from build123d import *

# Parameters (mm, degrees)
SKETCH1_W                   = 736.6
SKETCH1_H                   = 596.9
BOSS_EXTRUDE1_DEPTH         = 0.127
SKETCH5_W                   = 31.75
SKETCH5_H                   = 76.2
BOSS_EXTRUDE2_DEPTH         = 0.127
SKETCH6_W                   = 6.35
SKETCH6_H                   = 444.5
CUT_EXTRUDE1_DEPTH          = 1.127
FILLET1_R                   = 6.35
F_0_257_DIAMETER_HOLE1_D    = 6.5278
F_1_4_0_25_DIAMETER_HOLE2_D = 6.35
CUT_EXTRUDE2_DEPTH          = 1.127


with BuildPart() as part:
    # Sketch1 → Boss-Extrude1 (new body)
    with BuildSketch(Plane.XY):
        Rectangle(SKETCH1_W, SKETCH1_H)
    extrude(amount=BOSS_EXTRUDE1_DEPTH)

    # Sketch5 → Boss-Extrude2 (add)
    with BuildSketch(Plane.XY.offset(0.127)):
        with Locations((-384.175, 260.35)):
            Rectangle(SKETCH5_W, SKETCH5_H)
        with Locations((-384.175, -260.35)):
            Rectangle(SKETCH5_W, SKETCH5_H)
    extrude(amount=-BOSS_EXTRUDE2_DEPTH)

    # Sketch6 → Cut-Extrude1 (cut, through all)
    with BuildSketch(Plane.XY.offset(0.127)):
        with Locations((-365.125, 0)):
            Rectangle(SKETCH6_W, SKETCH6_H)
    extrude(amount=-CUT_EXTRUDE1_DEPTH, mode=Mode.SUBTRACT)

    # Fillet1
    fillet1_edges = [part.edges().sort_by_distance(p)[0] for p in [
        (-361.95, 222.25, 0.0635),
        (-361.95, -222.25, 0.0635),
    ]]
    fillet(fillet1_edges, radius=FILLET1_R)

    # F (0.257) Diameter Hole1 (through all)
    with Locations(Plane.XY.offset(0.127)):
        with Locations((349.25, 247.65), (349.25, 196.85), (349.25, -196.85), (349.25, -247.65)):
            Hole(F_0_257_DIAMETER_HOLE1_D / 2)

    # 1/4 (0.25) Diameter Hole2 (through all)
    with Locations(Plane.XY.offset(0.127)):
        with Locations((-387.35, 260.35), (-361.95, 260.35), (-361.95, -241.3), (-387.35, -241.3)):
            Hole(F_1_4_0_25_DIAMETER_HOLE2_D / 2)

    # Sketch13 → Cut-Extrude2 (cut, through all)
    with BuildSketch(Plane.XY.offset(0.127)):
        with BuildLine():
            Line((368.3, 298.45), (342.9, 298.45))
            Line((342.9, 298.45), (342.9, 288.925))
            ThreePointArc((342.9, 288.925), (344.759871939, 284.434871939), (349.25, 282.575))
            Line((349.25, 282.575), (368.3, 282.575))
            Line((368.3, 282.575), (368.3, 298.45))
        make_face()
    extrude(amount=-CUT_EXTRUDE2_DEPTH, mode=Mode.SUBTRACT)


solid = part.part
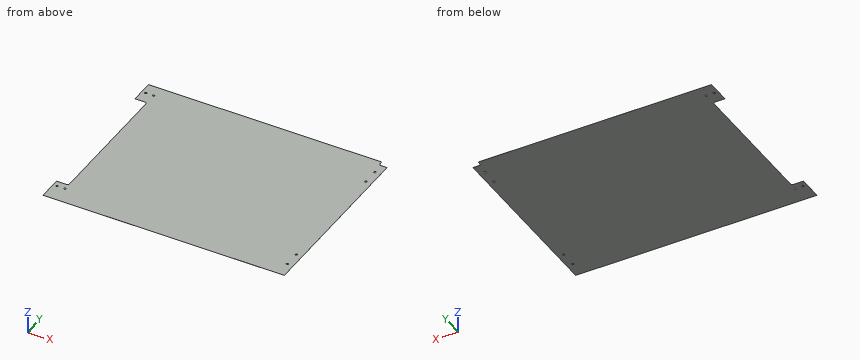
The model under review builds one solid part; all positions refer to its coordinate system, in mm. Round coordinates to 2 decimals unless told otherwise and drop trailing zeros. Write each loop counter-clockwise with the first axis right and the second up, starting at its lowest first coordinate (ties: lowest second). Pieces come first, ordered by that corner, then holes. Notation, with made-up numbers: (75.5, -13.5) - (86.5, -13.5) arc R6 cw to (86.5, -9.5) - close; hole circle Ø10 at (20, -4.75). An arc over 180 degrees is marked (long way). One line per item, written item: value. Start each with the question number.
1. Consider section B-B on y = 31. Write out the cut boundary in (x, z), and give its area (3 significant figures).
2. Consider section A-A on z = 0.05. State how many separate pieces and enclosed holes the cut face has, and give its area (3 significant figures).
3. Clearance check with a flat-ended pin moving along its axis: P1, Ø5.5, axis at x = -387.35, y = 260.35, coming from the +Z side. State where the tip first meets the part, or that it passes through.
4. To check wall thickness, follow L1, parallel to X at y = 260.35, z = 0.05 (3 decimals); L2, parallel to X at y = -247.65, z = 0.05; L3, parallel to X at y = 13.5, z = 0.05. State the ranges of each line that lie inside material, in increasing order. Write a range as from..to.
Checks:
1. outline: (-361.95, 0) - (368.3, 0) - (368.3, 0.13) - (-361.95, 0.13) - close
1. area: 92.7 mm^2
2. separate pieces: 1
2. enclosed holes: 8
2. area: 441,000 mm^2
3. P1: passes through
4. L1: x = -400.05..-390.525, -384.175..-365.125, -358.775..368.3
4. L2: x = -400.05..345.99, 352.51..368.3
4. L3: x = -361.95..368.3
